from build123d import *

# Parameters (mm, degrees)
F0_W     = 15
F0_H     = 10
F1_DEPTH = 2
F2_W     = 6
F2_H     = 1
F3_DEPTH = 25
F5_DEPTH = 25


with BuildPart() as f1:
    # F0 (on Top) → F1 (new body)
    with BuildSketch(Plane.XY):
        with Locations((7.5, -5)):
            Rectangle(F0_W, F0_H)
    extrude(amount=F1_DEPTH)

    # F2 (on Front) → F3 (cut)
    with BuildSketch(Plane.XZ):
        with Locations((4, 0.5)):
            Rectangle(F2_W, F2_H)
        with Locations((11, 0.5)):
            Rectangle(F2_W, F2_H)
    extrude(amount=F3_DEPTH, mode=Mode.SUBTRACT)

    # F4 (on face) → F5 (cut)
    with BuildSketch(Plane(origin=(0, 0, 0), x_dir=(0, -1, 0), z_dir=(-1, 0, 0))):
        Polygon((0, 3.5), (0, 2.235531), (0, 1), (1, 1), (1, 2), (2, 2), (2, 1), (3, 1), (3, 2), (4, 2), (4, 1), (5, 1), (5, 2), (6, 2), (6, 1), (7, 1), (7, 2), (8, 2), (8, 1), (9, 1), (9, 2), (10, 2), (10, 1), (10.680856, 1), (10.680856, 3.5), align=None)
    extrude(amount=-F5_DEPTH, mode=Mode.SUBTRACT)


solid = f1.part
Geometry: final body of the model. Coordinates: model frame, mm. A direction names the side the tool comes from. Coordinates: 2 decimals unless noted, no trailing zeros. Order: outer loops, then holes, each group sorted by start corner. A loop starts at its lowest first (then second) coordinate and runs counter-clockwise, first axis right, second up.
(1) Section query D-D (y = -5.5). Return the cut outline in (x, z), plus the area to 3 significant figures.
(2) Draft query along Y for faces 1 (the face through (7.5, 0, 0.5)), 2 (the face through (7.5, -0.5, 1)), 3 (the face through (7.5, -4.5, 1)). Return one class per face: pulls with the +Y half, pulls with the -Y half, needs draft (parallel to the pull), parting line crosses it, or undercut.
(3) Access query for faces 4 (the face through (4, -3.5, 1)), 5 (the face through (7.5, -4.9, 0)), 6 (the face through (14.5, -8.5, 1)), 7 (the face through (14.5, -0.5, 1)). Directions: +Z, -Z, +X, -X, +Y, -Y. A direction counts if a zero-diameter tool reaches every point of the face in a straight line with its end or side. Return the directions, or none.
(4) Section query B-B (z = 1.3). Return the cut outline in (x, y), plus the area to 3 significant figures.
(5) First-contact query: pin 1 (0.8 mm diameter, centred on x = 4.5, y = -9.5, fed in from -Z); pin 2 (1.1 mm diameter, centred on x = 11, z = 1.5, fed in from +Y). Flat tips, straight axial feed; report the tip coordinate or a pass-through.
(6) Section query C-C (x = 2). Return the cut outline in (y, z), plus the area to 3 significant figures.
(7) Material intervals for probe 1 along X at (y, z) = (-8.5, 0.7); probe 2 along Y at (x, z) = (9, 1.6); probe 3 along Z at (x, y) = (9, -9.25), sorted ascending.
(8) Section query A-A (y = -0.75). Return the cut outline in (x, z), plus the area to 3 significant figures.
Solution:
1. outline: (0, 0) - (1, 0) - (1, 1) - (7, 1) - (7, 0) - (8, 0) - (8, 1) - (14, 1) - (14, 0) - (15, 0) - (15, 2) - (0, 2) - close
1. area: 18.0 mm2
2. face 1: pulls with the +Y half
2. face 2: needs draft
2. face 3: undercut
3. face 4: -Z, +Y, -Y
3. face 5: -Z, +X, -X, +Y, -Y
3. face 6: +Z, +X, -X
3. face 7: +Z, +X, -X, +Y
4. outline: (0, -10) - (15, -10) - (15, -9) - (0, -9) - close; (0, -8) - (15, -8) - (15, -7) - (0, -7) - close; (0, -6) - (15, -6) - (15, -5) - (0, -5) - close; (0, -4) - (15, -4) - (15, -3) - (0, -3) - close; (0, -2) - (15, -2) - (15, -1) - (0, -1) - close
4. area: 75.0 mm2
5. pin 1: stops at z = 1
5. pin 2: stops at y = -1
6. outline: (-10, 1) - (-9, 1) - (-9, 2) - (-10, 2) - close; (-8, 1) - (-7, 1) - (-7, 2) - (-8, 2) - close; (-6, 1) - (-5, 1) - (-5, 2) - (-6, 2) - close; (-4, 1) - (-3, 1) - (-3, 2) - (-4, 2) - close; (-2, 1) - (-1, 1) - (-1, 2) - (-2, 2) - close
6. area: 5.00 mm2
7. probe 1: x = 0 to 1, 7 to 8, 14 to 15
7. probe 2: y = -10 to -9, -8 to -7, -6 to -5, -4 to -3, -2 to -1
7. probe 3: z = 1 to 2
8. outline: (0, 0) - (1, 0) - (1, 1) - (0, 1) - close; (7, 0) - (8, 0) - (8, 1) - (7, 1) - close; (14, 0) - (15, 0) - (15, 1) - (14, 1) - close
8. area: 3.00 mm2
